Design review of the part built by this model. Coordinates are the model's own, in mm. Coordinates: 2 decimals unless noted, no trailing zeros. Order: outer loops, then holes, each group sorted by start corner. A loop starts at its lowest first (then second) coordinate and runs counter-clockwise, first axis right, second up. Notation, with made-up numbers: M -30,-14 L -15,-14 A29 ccw -15,13 Z; hole C 80,44 d5. An arc over 180 degrees is marked long. Use CSV: the item, a comma, the result in double quotes.
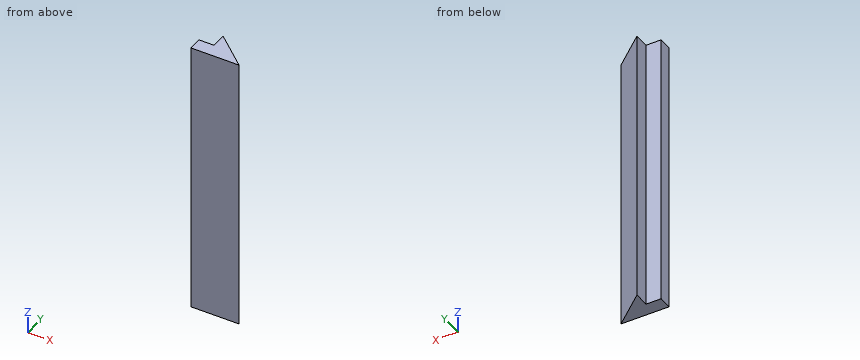
Autodesk Inventor part; units mm, degrees
ref_plane "YZ Plane" through (0, 0, 0) normal (1, 0, 0) x (0, 1, 0)
ref_plane "XZ Plane" through (0, 0, 0) normal (0, 1, 0) x (-1, 0, 0)
ref_plane "XY Plane" through (0, 0, 0) normal (0, 0, 1) x (1, 0, 0)
sketch "Sketch1" plane through (0, 0, 0) normal (0, 1, 0) x (-1, 0, 0)
  line L0 (12.2947, 115.8176) -> (-13.1053, 115.8176)
  line L1 (-13.1053, 115.8176) -> (-13.1053, -31.6824)
  line L2 (-13.1053, -31.6824) -> (12.2947, -31.6824)
  line L3 (12.2947, -31.6824) -> (12.2947, 115.8176)
  point P0 (0, 0)
  dimension "d0" = 25.4
  dimension "d1" = 147.5
extrude "Extrusion1" add sketch "Sketch1" along normal blind 15
sketch "Sketch2" plane through (-12.2947, 0, 115.8176) normal (0, 0, 1) x (1, 0, 0)
  line L0 (0, 15) -> (8, 15)
  line L1 (8, 15) -> (8, 7)
  line L2 (8, 7) -> (0, 7)
  line L3 (0, 7) -> (0, 15)
  point P0 (12.2947, 0)
  dimension "d13" = 8
extrude "Extrusion2" cut sketch "Sketch2" against normal through all
ref_plane "Work Plane1" through (-4.2947, 15, 78.9426) normal (0.6561, 0.7547, 0) x (0, 0, 1)
sketch "Sketch3" plane through (-4.2947, 15, 78.9426) normal (0.6561, 0.7547, 0) x (0, 0, 1)
  line L0 (36.875, 0) -> (36.875, 13.1319) construction
  line L1 (-110.625, 22.9728) -> (-110.625, 3.8032) construction
  line L2 (36.875, 0) -> (-110.625, 0)
  line L3 (-110.625, 0) -> (-110.625, 22.9728)
  line L4 (-110.625, 22.9728) -> (36.875, 22.9728)
  line L5 (36.875, 22.9728) -> (36.875, 0)
  point P0 (-78.9426, 13.0821)
extrude "Extrusion3" add sketch "Sketch3" along normal blind 15
sketch "Sketch4" plane through (5.5462, 26.3206, 78.9426) normal (0.6561, 0.7547, 0) x (0.7547, -0.6561, 0)
  line L0 (22.8638, 110.625) -> (22.8638, -36.875) construction
  line L1 (0, -36.875) -> (22.8638, -36.875)
  line L2 (-1.723, -37.6113) -> (24.2555, -37.6113)
  line L3 (24.2555, -37.6113) -> (24.2555, 112.242)
  line L4 (24.2555, 112.242) -> (-1.723, 112.242)
  line L5 (-1.723, 112.242) -> (-1.723, -37.6113)
extrude "Extrusion4" cut sketch "Sketch4" against normal blind 15
ref_plane "Work Plane2" through (-12.2947, 7, 42.0676) normal (-0.5, -0.866, 0) x (0, 0, -1)
sketch "Sketch5" plane through (-12.2947, 7, 42.0676) normal (-0.5, -0.866, 0) x (0, 0, -1)
  point P0 (42.0676, 14.1475)
properties part number "Ramp version 2 {needs editing}"
(1) Clearance check with flat-ended pins moving along their axes: P1, Ø10, axis at x = 8.5, z = 98.5, coming from the -Y side; P2, Ø9, axis at x = -9, z = 35.5, coming from the +Y side; P3, Ø6.5, axis at y = 11, z = 77, coming from the -X side; P4, Ø1.5, axis at x = -1, z = 63.5, coming from the +Y side. State where each tip first meets the part, or that it passes through.
The answers:
P1,"stops at y = 0"
P2,"stops at y = 7"
P3,"stops at x = -4.29"
P4,"stops at y = 12.79"
(2) Wall thickness on probe 1 along Y at (x, z) = (-10.5, 18.5); probe 2 along Y at (x, z) = (-1.25, -4.5); probe 3 along X at (y, z) = (6.25, 87): over which ranges is each line inside the solid? List them lowest first.
The answers:
probe 1,"y = 0 to 7"
probe 2,"y = 0 to 12.35"
probe 3,"x = -12.29 to 5.77"
(3) Add section C-C on x = -2. State the section outline as (y, z) points, and give its area (3 significant figures).
The answers:
outline,"M 0,-31.68 L 13,-31.68 L 13,115.82 L 0,115.82 Z"
area,"1,920 mm2"
(4) Add section A-A on z = 8. State the section outline as (x, y) points.
The answers:
outline,"M -12.29,0 L 12.96,0 L -4.29,15 L -4.29,7 L -12.29,7 Z"
(5) Add section B-B on y = 2.5. State the section outline as (x, z) points.
The answers:
outline,"M -12.29,-31.68 L 10.08,-31.68 L 10.08,115.82 L -12.29,115.82 Z"
